The model under review builds one solid part; all positions refer to its coordinate system, in mm. A direction names the side the tool comes from. Give positions to 0.01 mm unless a question says otherwise; leave off trailing zeros. Loops run counter-clockwise (first coordinate to the right, second up) from the corner with the lowest first, then second, coordinate; pieces in that order, holes last. Notation, with made-up numbers: M 42,57.5 L 74,57.5 A25 ccw 74,79.5 Z; hole C 84.5,29 d4. An arc over 180 degrees is marked long. Write item = value, one per line. Start each with the question number.
1. For pin 1 (2 mm diameter, centred on x = 5.5, y = -5.5, fed in from +Z); pin 2 (4 mm diameter, centred on x = 0.5, z = 50, fed in from -Y); pin 3 (1.7 mm diameter, centred on x = -0.5, z = 50, fed in from +Y); pin 4 (1 mm diameter, centred on x = 5.5, z = 8, fed in from +Y), all flat-tipped, find the tip position at first contact; note any pin that passes through.
2. For faces 4 (the face through (-0.867, -3.905, 22.692)), 5 (the face through (3, -3, 53)), 6 (the face through (-2.78, 1.63, 52.76)), list the 3-axis set-ups (+Z, -Z, +X, -X, +Y, -Y) from which the entire face can be reached by the end or side of a thin tool; tool diameter is ignored.
3. We need section B-B on z = 33.5. Give the boundary of the cut face in (x, y).
4. Draft analysis for pull direction Y (two halves, no side actions). For faces 1 (the face through (-5.158, -3.955, 49.255)), 2 (the face through (-2.808, -1.594, 52.765)), 3 (the face through (4, 2, 45)), state which applies: pulls with the +Y half, pulls with the -Y half, needs draft (parallel to the pull), parting line crosses it, or undercut.
5. We need section A-A on x = 0. Give the boundary of the cut face in (y, z).
6. Wall thickness on line 1 along Z through (x, y) = (-1, -2); line 2 along X through (y, z) = (-2, 26); line 3 along Z through (x, y) = (1.5, -4): over which ranges is each line inside the solid? List them lowest first. Write a range as from..to.
from build123d import *

# Parameters (mm, degrees)
SCHIZZO1_R                   = 4
ESTRUSIONE_ESTRUSIONE1_DEPTH = 45
SMUSSO1_SIZE                 = 1
SCHIZZO6_R                   = 6.5
ESTRUSIONE_ESTRUSIONE3_DEPTH = 8
TAGLIO_ESTRUSIONE3_DEPTH     = 6
SCHIZZO8_R                   = 3.464101615
TAGLIO_ESTRUSIONE4_DEPTH     = 1
TAGLIO_ESTRUSIONE4_TAPER     = 45
RACCORDO1_R                  = 0.5
SCHIZZO9_R                   = 8
SCHIZZO9_R_2                 = 6.5
ESTRUSIONE_ESTRUSIONE4_DEPTH = 1
RACCORDO2_R                  = 0.1


with BuildPart() as part:
    # Schizzo1 → Estrusione-Estrusione1 (new body)
    with BuildSketch(Plane.XY):
        Circle(SCHIZZO1_R)
    extrude(amount=ESTRUSIONE_ESTRUSIONE1_DEPTH)

    # Smusso1
    smusso1_edges = [part.edges().sort_by_distance(p)[0] for p in [
        (-4, 0, 0),
    ]]
    chamfer(smusso1_edges, length=SMUSSO1_SIZE)

    # Schizzo6 → Estrusione-Estrusione3 (add)
    with BuildSketch(Plane.XY.offset(45)):
        Circle(SCHIZZO6_R)
    extrude(amount=ESTRUSIONE_ESTRUSIONE3_DEPTH)

    # Schizzo7 → Taglio-Estrusione3 (cut)
    with BuildSketch(Plane.XY.offset(53)):
        Polygon((1.732050808, 3), (-1.732050808, 3), (-3.464101615, 0), (-1.732050808, -3), (1.732050808, -3), (3.464101615, 0), align=None)
    extrude(amount=-TAGLIO_ESTRUSIONE3_DEPTH, mode=Mode.SUBTRACT)

    # Schizzo8 → Taglio-Estrusione4 (cut)
    with BuildSketch(Plane.XY.offset(53)):
        Circle(SCHIZZO8_R)
    extrude(amount=-TAGLIO_ESTRUSIONE4_DEPTH, taper=TAGLIO_ESTRUSIONE4_TAPER, mode=Mode.SUBTRACT)

    # Raccordo1
    raccordo1_edges = [part.edges().sort_by_distance(p)[0] for p in [
        (-6.5, 0, 53),
    ]]
    fillet(raccordo1_edges, radius=RACCORDO1_R)

    # Schizzo9 → Estrusione-Estrusione4 (add)
    with BuildSketch(Plane(origin=(0, 0, 45), x_dir=(-1, 0, 0), z_dir=(0, 0, -1))):
        Circle(SCHIZZO9_R)
        Circle(SCHIZZO9_R_2, mode=Mode.SUBTRACT)
    extrude(amount=-ESTRUSIONE_ESTRUSIONE4_DEPTH)

    # Raccordo2
    raccordo2_edges = [part.edges().sort_by_distance(p)[0] for p in [
        (-6.5, 0, 46),
        (8, 0, 46),
        (8, 0, 45),
    ]]
    fillet(raccordo2_edges, radius=RACCORDO2_R)


solid = part.part
Final values:
q1.pin_1 = 46
q1.pin_2 = -6.5
q1.pin_3 = 6.5
q1.pin_4 = through
q2.face_4 = -Z
q2.face_5 = +Z, +X, -X, +Y, -Y
q2.face_6 = +Z
q3.outline = C 0,0 d8
q4.face_1 = parting line crosses it
q4.face_2 = undercut
q4.face_3 = needs draft
q5.outline = M -8,45.1 A0.1 ccw -7.9,45 L -4,45 L -4,1 L -3,0 L 3,0 L 4,1 L 4,45 L 7.9,45 A0.1 ccw 8,45.1 L 8,45.9 A0.1 ccw 7.9,46 L 6.6,46 A0.1 cw 6.5,46.1 L 6.5,52.5 A0.5 ccw 6,53 L 3.46,53 L 3,52.54 L 3,47 L -3,47 L -3,52.54 L -3.46,53 L -6,53 A0.5 ccw -6.5,52.5 L -6.5,46.1 A0.1 cw -6.6,46 L -7.9,46 A0.1 ccw -8,45.9 Z
q6.line_1 = 0..47
q6.line_2 = -3.46..3.46
q6.line_3 = 45..53
